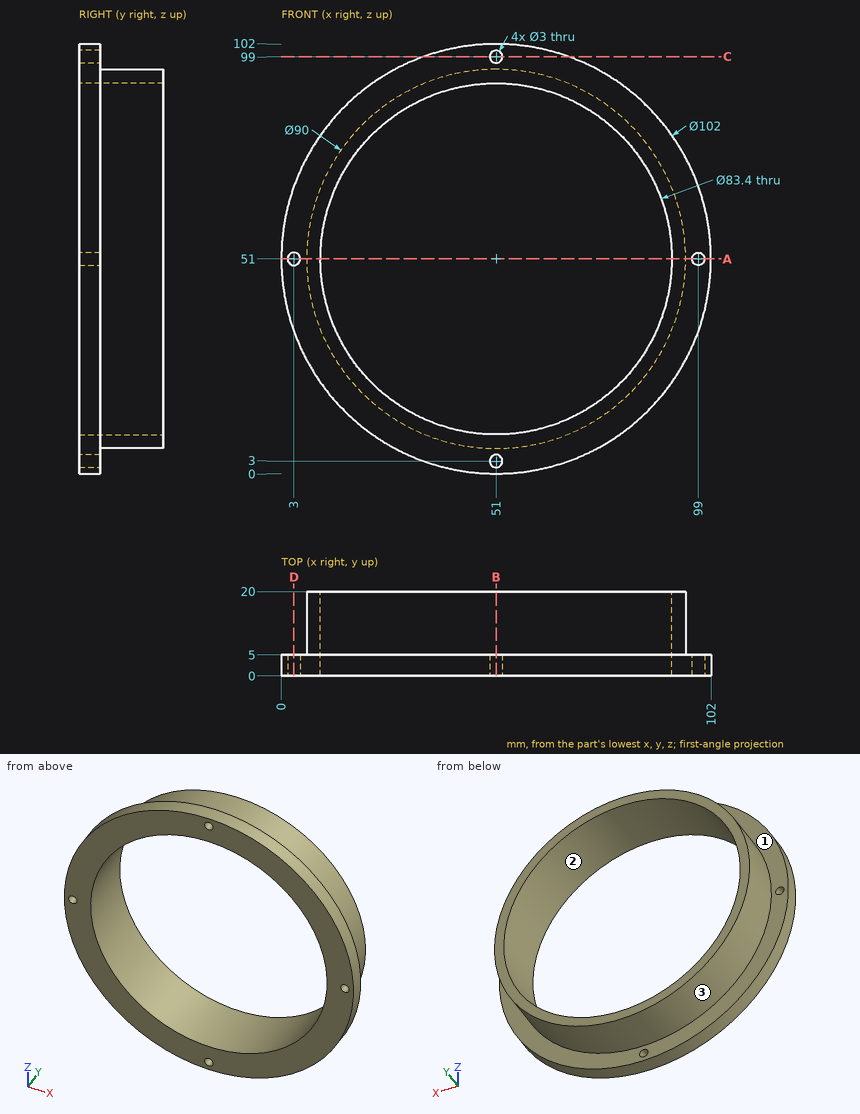
Drawing for the job (mm, zero at the part's lowest x, y, z). Round coordinates to 2 decimals unless told otherwise and drop trailing zeros. Loops run counter-clockwise (first coordinate to the right, second up) from the corner with the lowest first, then second, coordinate; pieces in that order, holes last. Notation, with made-up numbers: (57, 40) -> (101, 40) arc R24 cw to (101, 50) -> close; hole circle Ø4 at (-4, 3.5). An arc over 180 degrees is marked (long way). Use one line per item in the form item = value. Start each with the question number.
Item 1: Drop flat-ended pins along their axis: pin 1 Ø3 at (x, y) = (62.5, 6) entering from -Z; pin 2 Ø8 at (y, z) = (10.5, 65.5) entering from +X; pin 3 Ø1.5 at (x, y) = (13.5, 14) entering from +Z. Give the stop position or say it passes through.
Item 2: Band-saw the part on C-C (z = 99). List the corners of the cut face in (x, y), plus the area to 3 significant figures.
Item 3: Drill centre lines: line 1 along X through (y, z) = (8.75, 51); line 2 along Z through (x, y) = (43, 2); line 3 along Z through (x, y) = (68.5, 18.5). Where is each one in solid material? Low to high.
Item 4: Band-saw the part on B-B (x = 51). List the corners of the cut face in (y, z), plus the area to 3 significant figures.
Item 5: Two-plate mould, pull along Z, no slides. Class the marked faces 1, 2 and 3: released by +Z, released by -Z, zero draft, split by the parting line, or undercut.
Item 6: Band-saw the part on A-A (z = 51). List the corners of the cut face in (x, y).
Item 7: Band-saw the part on D-D (x = 3). List the corners of the cut face in (y, z), plus the area to 3 significant figures.
Data:
q1.pin_1 = 1.07
q1.pin_2 = 94.76
q1.pin_3 = 76.97
q2.outline = (33.77, 0) -> (49.5, 0) -> (49.5, 5) -> (33.77, 5) -> close; (52.5, 0) -> (68.23, 0) -> (68.23, 5) -> (52.5, 5) -> close
q2.area = 157 mm^2
q3.line_1 = 6 to 9.3, 92.7 to 96
q3.line_2 = 0.63 to 10.07, 91.93 to 101.37
q3.line_3 = 9.54 to 13.15, 88.85 to 92.46
q4.outline = (0, 0) -> (5, 0) -> (5, 1.5) -> (0, 1.5) -> close; (0, 4.5) -> (5, 4.5) -> (5, 6) -> (20, 6) -> (20, 9.3) -> (0, 9.3) -> close; (0, 92.7) -> (20, 92.7) -> (20, 96) -> (5, 96) -> (5, 97.5) -> (0, 97.5) -> close; (0, 100.5) -> (5, 100.5) -> (5, 102) -> (0, 102) -> close
q4.area = 162 mm^2
q5.face_1 = zero draft
q5.face_2 = undercut
q5.face_3 = split by the parting line
q6.outline = (0, 0) -> (1.5, 0) -> (1.5, 5) -> (0, 5) -> close; (4.5, 0) -> (9.3, 0) -> (9.3, 20) -> (6, 20) -> (6, 5) -> (4.5, 5) -> close; (92.7, 0) -> (97.5, 0) -> (97.5, 5) -> (96, 5) -> (96, 20) -> (92.7, 20) -> close; (100.5, 0) -> (102, 0) -> (102, 5) -> (100.5, 5) -> close
q7.outline = (0, 33.77) -> (5, 33.77) -> (5, 49.5) -> (0, 49.5) -> close; (0, 52.5) -> (5, 52.5) -> (5, 68.23) -> (0, 68.23) -> close
q7.area = 157 mm^2
